The drawing under review shows one solid part. Ordinate dimensions are in mm from its lowest x, y, z. A direction names the side the tool comes from. Coordinates: 2 decimals unless noted, no trailing zeros. Order: outer loops, then holes, each group sorted by start corner. A loop starts at its lowest first (then second) coordinate and runs counter-clockwise, first axis right, second up. Notation, with made-up numbers: (-27.75, -39) - (-23.75, -39) arc R24 cw to (-23.75, -28) - close; hole circle Ø5 at (-38.75, -7). An arc over 180 degrees is marked (long way). Answer in a Markdown table with one row per item.
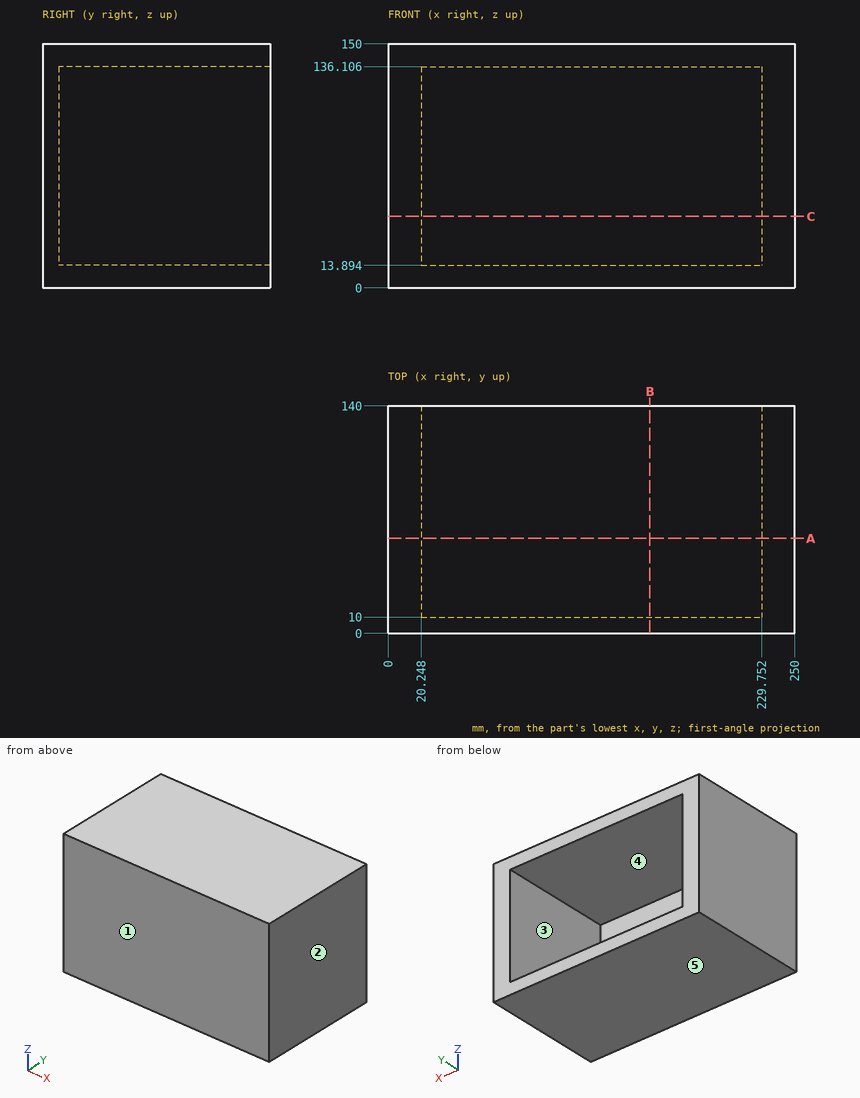
Item 1: Tool access review of the marked faces 4 and 5: name each direction out of +Z, -Z, +X, -X, +Y, -Y from which nothing blocks a thin tool from reaching the whole face with its end or side.
Check values:
| item | result |
|---|---|
| face 4 | +Y |
| face 5 | -Z, +X, -X, +Y, -Y |
Item 2: Mouldability with a two-part tool opening along X and no side actions: class the marked faces 1, 2 and 3 as +X half, -X half, draft (parallel to the pull), parting line (faces both ways), or undercut.
Check values:
| item | result |
|---|---|
| face 1 | draft |
| face 2 | +X half |
| face 3 | undercut |
Item 3: We need section A-A, the plane y = 58.5. Write out the cut boundary in (x, z) (1 decimal).
Check values:
| item | result |
|---|---|
| outline | (0, 0) - (250, 0) - (250, 150) - (0, 150) - close; hole (20.2, 13.9) - (229.8, 13.9) - (229.8, 136.1) - (20.2, 136.1) - close |
Item 4: We need section C-C, the plane z = 44. Write out the cut boundary in (x, y).
Check values:
| item | result |
|---|---|
| outline | (0, 0) - (250, 0) - (250, 140) - (229.75, 140) - (229.75, 10) - (20.25, 10) - (20.25, 140) - (0, 140) - close |
Item 5: We need section B-B, the plane x = 161. Write out the cut boundary in (y, z) (1 decimal).
Check values:
| item | result |
|---|---|
| outline | (0, 0) - (140, 0) - (140, 13.9) - (10, 13.9) - (10, 136.1) - (140, 136.1) - (140, 150) - (0, 150) - close |
Item 6: To check wall thickness, follow line 1 (X direction, y = 50.5, z = 17); line 2 (Z direction, x = 58, y = 111.5) (1 decimal); line 3 (Y direction, x = 132.5, z = 111.5). State the ranges of each line that lie inside material, in increasing order. Write a range as from..to.
Check values:
| item | result |
|---|---|
| line 1 | 0..20.25, 229.75..250 |
| line 2 | 0..13.9, 136.1..150 |
| line 3 | 0..10 |
